from build123d import *

# Parameters (mm, degrees)
BOSS_EXTRUDE1_DEPTH     = 6.35
CUT_EXTRUDE1_DEPTH      = 7.3500001
CUT_EXTRUDE1_DEPTH_BACK = 4.175
CUT_EXTRUDE3_DEPTH      = 7.3500001
CUT_EXTRUDE3_DEPTH_BACK = 4.175


with BuildPart() as part:
    # Sketch1 → Revolve1 (revolve)
    with BuildSketch(Plane.XY):
        with BuildLine():
            Line((0, 0), (30.1625, 0))
            ThreePointArc((30.1625, 0), (31.285032015, 0.464967985), (31.75, 1.5875))
            Line((31.75, 1.5875), (31.75, 7.9375))
            ThreePointArc((31.75, 7.9375), (31.285032015, 9.060032015), (30.1625, 9.525))
            Line((30.1625, 9.525), (25.4, 9.525))
            Line((25.4, 9.525), (25.4, 3.175))
            Line((25.4, 3.175), (0, 3.175))
            Line((0, 3.175), (0, 0))
        make_face()
    revolve(axis=Axis((0, 3.175, 0), (0, -1, 0)))

    # Sketch2 → Boss-Extrude1 (add)
    with BuildSketch(Plane(origin=(0, 3.175, 0), x_dir=(1, 0, 0), z_dir=(0, 1, 0))):
        Polygon((0, -5.499261314), (4.7625, -2.749630657), (4.7625, 2.749630657), (0, 5.499261314), (-4.7625, 2.749630657), (-4.7625, -2.749630657), align=None)
    extrude(amount=BOSS_EXTRUDE1_DEPTH)

    # Sketch3 → Cut-Extrude1 (cut, two sides)
    with BuildSketch(Plane(origin=(0, 3.175, 0), x_dir=(1, 0, 0), z_dir=(0, 1, 0))) as cut_extrude1_sk:
        Polygon((-20.156339589, -4.7625), (-21.915105149, -4.7625), (-21.915105149, 2.597727273), (-22.418122878, 2.597727273), (-22.418122878, 4.356492833), (-21.333041777, 4.7625), (-20.156339589, 4.7625), align=None)
        Polygon((-14.001558374, -3.767243493), (-15.129755281, -4.7625), (-18.185587986, -4.7625), (-19.313784892, -3.767243493), (-19.313784892, 3.761854017), (-18.198163429, 4.7625), (-15.1477202, 4.7625), (-14.019523293, 3.761854017), (-14.019523293, 2.288730668), (-15.783678329, 2.288730668), (-15.783678329, 3.00373444), (-17.555019332, 3.00373444), (-17.555019332, 0.882077518), (-15.129755281, 0.882077518), (-14.001558374, -0.105993022), align=None)
        Polygon((-7.769528008, -3.767243493), (-8.895928423, -4.7625), (-11.928406733, -4.7625), (-13.05660364, -3.767243493), (-13.05660364, -2.234835911), (-11.340953885, -2.234835911), (-11.340953885, -3.00373444), (-9.526497077, -3.00373444), (-9.526497077, -0.882077518), (-11.98230149, -0.882077518), (-13.105108921, 0.113178989), (-13.105108921, 3.761854017), (-11.98230149, 4.7625), (-8.908503866, 4.7625), (-7.769528008, 3.756464542), align=None)
        Polygon((9.877353766, 3.175), (11.051442308, 3.175), (11.051442308, -3.175), (10.481570513, -3.175), (10.481570513, 2.523717949), (9.504647436, 2.523717949), align=None)
        Polygon((16.750160256, 3.337820513), (14.094150641, -4.070512821), (13.49375, -4.070512821), (16.149759615, 3.337820513), align=None)
        Polygon((20.704917869, 3.337820513), (20.820673077, 3.337820513), (20.820673077, -1.058333333), (21.553365385, -1.058333333), (21.553365385, -1.709615385), (20.820673077, -1.709615385), (20.820673077, -3.175), (20.250801282, -3.175), (20.250801282, -1.709615385), (17.238621795, -1.709615385), align=None)
    extrude(amount=CUT_EXTRUDE1_DEPTH, mode=Mode.SUBTRACT)
    extrude(cut_extrude1_sk.sketch, amount=-CUT_EXTRUDE1_DEPTH_BACK, mode=Mode.SUBTRACT)

    # Sketch4 → Cut-Extrude3 (cut, two sides)
    with BuildSketch(Plane(origin=(0, 3.175, 0), x_dir=(1, 0, 0), z_dir=(0, 1, 0))) as cut_extrude3_sk:
        with BuildLine():
            Line((-20.897368408, 6.35), (-15.805631592, 6.35))
            Line((-15.805631592, 6.35), (-13.589, 7.629772846))
            Line((-13.589, 7.629772846), (-13.589, 13.12903416))
            Line((-13.589, 13.12903416), (-17.108932059, 15.161267882))
            ThreePointArc((-17.108932059, 15.161267882), (-19.892207199, 11.264088635), (-21.802466353, 6.872558542))
            Line((-21.802466353, 6.872558542), (-20.897368408, 6.35))
        make_face()
        with BuildLine():
            ThreePointArc((-7.4295, 21.619022405), (-11.544244404, 19.730940706), (-15.206214659, 17.068996331))
            Line((-15.206214659, 17.068996331), (-12.192, 15.328738686))
            Line((-12.192, 15.328738686), (-7.4295, 18.078369343))
            Line((-7.4295, 18.078369343), (-7.4295, 21.619022405))
        make_face()
        Polygon((-8.705368408, 6.35), (-3.613631592, 6.35), (-1.397, 7.629772846), (-1.397, 13.12903416), (-6.1595, 15.878664817), (-10.922, 13.12903416), (-10.922, 7.629772846), align=None)
        with BuildLine():
            ThreePointArc((4.7625, 22.358403202), (0, 22.86), (-4.7625, 22.358403202))
            Line((-4.7625, 22.358403202), (-4.7625, 18.078369343))
            Line((-4.7625, 18.078369343), (0, 15.328738686))
            Line((0, 15.328738686), (4.7625, 18.078369343))
            Line((4.7625, 18.078369343), (4.7625, 22.358403202))
        make_face()
        Polygon((1.27, 7.629772846), (3.486631592, 6.35), (8.578368408, 6.35), (10.795, 7.629772846), (10.795, 13.12903416), (6.0325, 15.878664817), (1.27, 13.12903416), align=None)
        with BuildLine():
            Line((12.192, 15.328738686), (15.206214659, 17.068996331))
            ThreePointArc((15.206214659, 17.068996331), (11.544244404, 19.730940706), (7.4295, 21.619022405))
            Line((7.4295, 21.619022405), (7.4295, 18.078369343))
            Line((7.4295, 18.078369343), (12.192, 15.328738686))
        make_face()
        with BuildLine():
            Line((13.462, 7.629772846), (15.678631592, 6.35))
            Line((15.678631592, 6.35), (20.770368408, 6.35))
            Line((20.770368408, 6.35), (21.782830062, 6.934545009))
            ThreePointArc((21.782830062, 6.934545009), (19.860135036, 11.320540463), (17.065866333, 15.209727358))
            Line((17.065866333, 15.209727358), (13.462, 13.12903416))
            Line((13.462, 13.12903416), (13.462, 7.629772846))
        make_face()
        with BuildLine():
            Line((20.650522628, -6.35), (15.798477372, -6.35))
            Line((15.798477372, -6.35), (13.462, -7.69896584))
            Line((13.462, -7.69896584), (13.462, -13.198227154))
            Line((13.462, -13.198227154), (17.025077395, -15.255370847))
            ThreePointArc((17.025077395, -15.255370847), (19.829723184, -11.373727554), (21.764149656, -6.992952864))
            Line((21.764149656, -6.992952864), (20.650522628, -6.35))
        make_face()
        with BuildLine():
            ThreePointArc((7.4295, -21.619022405), (11.544244404, -19.730940706), (15.206214659, -17.068996331))
            Line((15.206214659, -17.068996331), (12.192, -15.328738686))
            Line((12.192, -15.328738686), (7.4295, -18.078369343))
            Line((7.4295, -18.078369343), (7.4295, -21.619022405))
        make_face()
        Polygon((8.458522628, -6.35), (3.606477372, -6.35), (1.27, -7.69896584), (1.27, -13.198227154), (6.0325, -15.947857811), (10.795, -13.198227154), (10.795, -7.69896584), align=None)
        with BuildLine():
            Line((-4.7625, -18.078369343), (-4.7625, -22.358403202))
            ThreePointArc((-4.7625, -22.358403202), (0, -22.86), (4.7625, -22.358403202))
            Line((4.7625, -22.358403202), (4.7625, -18.078369343))
            Line((4.7625, -18.078369343), (0, -15.328738686))
            Line((0, -15.328738686), (-4.7625, -18.078369343))
        make_face()
        Polygon((-1.397, -7.69896584), (-3.733477372, -6.35), (-8.585522628, -6.35), (-10.922, -7.69896584), (-10.922, -13.198227154), (-6.1595, -15.947857811), (-1.397, -13.198227154), align=None)
        with BuildLine():
            Line((-12.192, -15.328738686), (-15.206214659, -17.068996331))
            ThreePointArc((-15.206214659, -17.068996331), (-11.544244404, -19.730940706), (-7.4295, -21.619022405))
            Line((-7.4295, -21.619022405), (-7.4295, -18.078369343))
            Line((-7.4295, -18.078369343), (-12.192, -15.328738686))
        make_face()
        with BuildLine():
            Line((-13.589, -7.69896584), (-15.925477372, -6.35))
            Line((-15.925477372, -6.35), (-20.777522628, -6.35))
            Line((-20.777522628, -6.35), (-21.783940581, -6.931055676))
            ThreePointArc((-21.783940581, -6.931055676), (-19.861945981, -11.317362848), (-17.068296652, -15.207000013))
            Line((-17.068296652, -15.207000013), (-13.589, -13.198227154))
            Line((-13.589, -13.198227154), (-13.589, -7.69896584))
        make_face()
    extrude(amount=CUT_EXTRUDE3_DEPTH, mode=Mode.SUBTRACT)
    extrude(cut_extrude3_sk.sketch, amount=-CUT_EXTRUDE3_DEPTH_BACK, mode=Mode.SUBTRACT)


solid = part.part
Read the model definition and answer for the solid it produces. Units are mm, in the model's axes. A direction names the side the tool comes from. Coordinates: 2 decimals unless noted, no trailing zeros. Write each loop counter-clockwise with the first axis right and the second up, starting at its lowest first coordinate (ties: lowest second). Pieces come first, ordered by that corner, then holes. Notation, with made-up numbers: M 58,22.5 L 79,22.5 A19 cw 79,28.5 Z; hole C -15,34 d1. An arc over 180 degrees is marked long. Use a Markdown table: item, result.
Q1. The part is cut by section B-B, the plane x = 2. Give the number of separate pieces and of enclosed holes in the cut face, then the cut area to 3 significant figures.
Answer block:
| item | result |
|---|---|
| separate pieces | 5 |
| enclosed holes | 0 |
| area | 255 mm2 |
Q2. The part is cut by section A-A, the plane y = 6.5. Write down the section's boundary in (x, z).
Answer block:
| item | result |
|---|---|
| outline | C 0,0 d63.5; M -4.76,-2.75 L 0,-5.5 L 4.76,-2.75 L 4.76,2.75 L 0,5.5 L -4.76,2.75 Z; hole C 0,0 d50.8 |
Q3. Straight lines are drawn through the part: L1, parallel to Z at x = 0, y = 7; L2, parallel to Z at x = 12.5, y = 1.5; L3, parallel to X at y = 8.5, z = -2.5. For each, find the intervals that lie inside material, in ascending order. Write a range as [from, to].
Answer block:
| item | result |
|---|---|
| L1 | z = [-31.75, -25.4], [-5.5, 5.5], [25.4, 31.75] |
| L2 | z = [-29.18, -19.14], [-15.51, 15.51], [19.14, 29.18] |
| L3 | x = [-31.55, -25.28], [-4.76, 4.76], [25.28, 31.55] |
Q4. Each of these flat-tipped pins is pushed along its axis until it touches: pin 1 Ø2.5 at (y, z) = (2, -20.5) entering from -X; pin 2 Ø4 at (x, z) = (-6.5, -4) entering from -Y; pin 3 Ø0.9 at (x, y) = (-17, 1) entering from -Z; pin 4 Ø1.5 at (x, y) = (-10, 1.5) entering from +Z. Where does it stop, or does it pass through?
Answer block:
| item | result |
|---|---|
| pin 1 | stops at x = -25.25 |
| pin 2 | stops at y = 0 |
| pin 3 | stops at z = -27.01 |
| pin 4 | stops at z = 30.37 |
Q5. Which of the six approach directions +Z, -Z, +X, -X, +Y, -Y give full straight-line access (tool end or side, diameter ignored) to faces 1 (the face through (20.251, 2, 2)), 2 (the face through (-4.762, 6, 0))?
Answer block:
| item | result |
|---|---|
| face 1 | +Y, -Y |
| face 2 | +Y |
